from build123d import *

# Parameters (mm, degrees)
F0_W     = 36.7
F0_H     = 23.3
F0_W_2   = 33.7
F0_H_2   = 20.3
F1_DEPTH = 95
F2_W     = 20.7
F2_H     = 79
F3_DEPTH = 23.301
F4_W     = 7.3
F4_H     = 79
F5_DEPTH = 36.701
F6_W     = 36.7
F6_H     = 23.3
F7_DEPTH = 1.5


with BuildPart() as f1:
    # F0 (on Top) → F1 (new body)
    with BuildSketch(Plane.XY):
        with Locations((16.85, 10.15)):
            Rectangle(F0_W, F0_H)
        with Locations((16.85, 10.15)):
            Rectangle(F0_W_2, F0_H_2, mode=Mode.SUBTRACT)
    extrude(amount=F1_DEPTH)

    # F2 (on face) → F3 (cut, through all)
    with BuildSketch(Plane(origin=(0, 21.8, 0), x_dir=(-1, 0, 0), z_dir=(0, 1, 0))):
        with Locations((-16.85, 47.5)):
            Rectangle(F2_W, F2_H)
    extrude(amount=-F3_DEPTH, mode=Mode.SUBTRACT)

    # F4 (on face) → F5 (cut, through all)
    with BuildSketch(Plane.YZ.offset(35.2)):
        with Locations((10.15, 47.5)):
            Rectangle(F4_W, F4_H)
    extrude(amount=-F5_DEPTH, mode=Mode.SUBTRACT)

    # F6 (on Top) → F7 (join)
    with BuildSketch(Plane.XY):
        with Locations((16.85, 10.15)):
            Rectangle(F6_W, F6_H)
    extrude(amount=-F7_DEPTH)


solid = f1.part
The model under review builds one solid part; all positions refer to its coordinate system, in mm. A direction names the side the tool comes from. Coordinates: 2 decimals unless noted, no trailing zeros. Write each loop counter-clockwise with the first axis right and the second up, starting at its lowest first coordinate (ties: lowest second). Pieces come first, ordered by that corner, then holes. Notation, with made-up numbers: (40.5, -31) -> (67.5, -31) arc R26 cw to (67.5, -4) -> close; hole circle Ø8 at (5.25, 88.5). An arc over 180 degrees is marked (long way). Answer in a Markdown table with one row per item.
1. Wall thickness on probe 1 along Y at (x, z) = (11, 3); probe 2 along X at (y, z) = (3.5, 90.5); probe 3 along Z at (x, y) = (5, 6.25): over which ranges is each line inside the solid? List them lowest first. Write a range as [from, to].
Answers below:
| item | result |
|---|---|
| probe 1 | y = [-1.5, 0], [20.3, 21.8] |
| probe 2 | x = [-1.5, 0], [33.7, 35.2] |
| probe 3 | z = [-1.5, 0] |
2. We need section D-D, the plane x = 16. State the section outline as (y, z) points, and give its area (4 significant figures).
Answers below:
| item | result |
|---|---|
| outline | (-1.5, -1.5) -> (21.8, -1.5) -> (21.8, 8) -> (20.3, 8) -> (20.3, 0) -> (0, 0) -> (0, 8) -> (-1.5, 8) -> close; (-1.5, 87) -> (0, 87) -> (0, 95) -> (-1.5, 95) -> close; (20.3, 87) -> (21.8, 87) -> (21.8, 95) -> (20.3, 95) -> close |
| area | 82.95 mm^2 |
3. For faces 4 (the flat face through (17, 10, -1.5)), 5 (the flat face through (28, 20.3, 47)), list the 3-axis set-ups (+Z, -Z, +X, -X, +Y, -Y) from which the entire face can be reached by the end or side of a thin tool; tool diameter is ignored.
Answers below:
| item | result |
|---|---|
| face 4 | -Z, +X, -X, +Y, -Y |
| face 5 | +Z |
4. Draft analysis for pull direction Y (two halves, no side actions). For faces 1 (the flat face through (15.4, -0.2, 95)), 2 (the flat face through (28, 0, 47)), 3 (the flat face through (4, -1.5, 47)), state which applies: +Y half, -Y half, draft (parallel to the pull), parting line (faces both ways), or undercut.
Answers below:
| item | result |
|---|---|
| face 1 | draft |
| face 2 | undercut |
| face 3 | -Y half |
5. We need section A-A, the plane y = 11.5. State the section outline as (x, z) points, and give its area (3 significant figures).
Answers below:
| item | result |
|---|---|
| outline | (-1.5, -1.5) -> (35.2, -1.5) -> (35.2, 8) -> (33.7, 8) -> (33.7, 0) -> (0, 0) -> (0, 8) -> (-1.5, 8) -> close; (-1.5, 87) -> (0, 87) -> (0, 95) -> (-1.5, 95) -> close; (33.7, 87) -> (35.2, 87) -> (35.2, 95) -> (33.7, 95) -> close |
| area | 103 mm^2 |
6. We need section C-C, the plane x = 2. State the section outline as (y, z) points.
Answers below:
| item | result |
|---|---|
| outline | (-1.5, -1.5) -> (21.8, -1.5) -> (21.8, 95) -> (20.3, 95) -> (20.3, 0) -> (0, 0) -> (0, 95) -> (-1.5, 95) -> close |
7. We need section B-B, the plane z = 40.5. State the section outline as (x, y) points.
Answers below:
| item | result |
|---|---|
| outline | (-1.5, -1.5) -> (6.5, -1.5) -> (6.5, 0) -> (0, 0) -> (0, 6.5) -> (-1.5, 6.5) -> close; (-1.5, 13.8) -> (0, 13.8) -> (0, 20.3) -> (6.5, 20.3) -> (6.5, 21.8) -> (-1.5, 21.8) -> close; (27.2, -1.5) -> (35.2, -1.5) -> (35.2, 6.5) -> (33.7, 6.5) -> (33.7, 0) -> (27.2, 0) -> close; (27.2, 20.3) -> (33.7, 20.3) -> (33.7, 13.8) -> (35.2, 13.8) -> (35.2, 21.8) -> (27.2, 21.8) -> close |
8. Clearance check with a flat-ended pin moving along its axis: pin 1 Ø10 at (x, y) = (11, 15) entering from +Z. State where the tip first meets the part, or that it passes through.
Answers below:
| item | result |
|---|---|
| pin 1 | stops at z = 0 |
